CAD build for the part. Positions are in the model's coordinates, mm. A direction names the side the tool comes from. Round coordinates to 2 decimals unless told otherwise and drop trailing zeros. Order: outer loops, then holes, each group sorted by start corner. A loop starts at its lowest first (then second) coordinate and runs counter-clockwise, first axis right, second up. Notation, with made-up numbers: M 66,34 L 97,34 A12 cw 97,40 Z; hole C 54.5,8.5 d5. An arc over 180 degrees is marked long. Put each result on its own line as item: value.
```python
from build123d import *

# Parameters (mm, degrees)
BOSS_EXTRUDE1_DEPTH = 127
SKETCH3_R           = 3.175
CUT_EXTRUDE1_DEPTH  = 145.837083045
SKETCH4_R           = 2.5
SKETCH4_R_2         = 2.413
SKETCH4_R_3         = 3.175
SKETCH4_R_4         = 4
CUT_EXTRUDE2_DEPTH  = 146.911891222


with BuildPart() as part:
    # Sketch2 → Boss-Extrude1 (new body)
    with BuildSketch(Plane.XY):
        Polygon((0, 0), (0, 50.8), (3.175, 50.8), (3.175, 3.175), (50.8, 3.175), (50.8, 0), align=None)
    extrude(amount=BOSS_EXTRUDE1_DEPTH)

    # Sketch3 → Cut-Extrude1 (cut, through all)
    with BuildSketch(Plane(origin=(0, 3.175, 0), x_dir=(1, 0, 0), z_dir=(0, 1, 0))):
        with Locations(Location((17.0942, -9.525, 0), (0, 0, 180))):
            Circle(SKETCH3_R)
        with Locations(Location((17.0942, -78.624999976, 0), (0, 0, 180))):
            Circle(SKETCH3_R)
        with Locations(Location((17.0942, -117.475, 0), (0, 0, 180))):
            Circle(SKETCH3_R)
    extrude(amount=-CUT_EXTRUDE1_DEPTH, mode=Mode.SUBTRACT)

    # Sketch4 → Cut-Extrude2 (cut, through all)
    with BuildSketch(Plane.ZY):
        with Locations((20.5994, 14.155)):
            Circle(SKETCH4_R)
        with Locations((9.525, 41.275)):
            Circle(SKETCH4_R_2)
        with Locations((67.7394, 14.155)):
            Circle(SKETCH4_R)
        with Locations((78.625, 41.275)):
            Circle(SKETCH4_R_2)
        with Locations((44.1706, 37.725)):
            Circle(SKETCH4_R_3)
        with Locations((94.9706, 37.725)):
            Circle(SKETCH4_R_4)
    extrude(amount=-CUT_EXTRUDE2_DEPTH, mode=Mode.SUBTRACT)


solid = part.part
```
Item 1: Probe line 1 along X through (y, z) = (16.5, 40) (3 decimals). List the from-to ranges inside material, lowest first. Write a range as [from, to].
Answers below:
line 1: [0, 3.175]
Item 2: Band-saw the part on C-C on y = 21.5. Give the cut face in (x, z) (3 decimals), and give its area (3 significant figures).
Answers below:
outline: M 0,0 L 3.175,0 L 3.175,127 L 0,127 Z
area: 403 mm²
Item 3: Band-saw the part on A-A on z = 95. Give the cut face in (x, y) (3 decimals), and give its area (3 significant figures).
Answers below:
outline: M 0,0 L 50.8,0 L 50.8,3.175 L 3.175,3.175 L 3.175,33.725 L 0,33.725 Z; M 0,41.725 L 3.175,41.725 L 3.175,50.8 L 0,50.8 Z
area: 287 mm²
Item 4: Mould opens along Y. For faces 1 (the flat face through (27, 3.175, 63)), 2 (the cylindrical face through (1.565, 16.263, 21.943)), 3 (the cylindrical face through (17.508, 1.61, 12.673)), 4 (the cylindrical face through (1.57, 43.31, 10.82)) say: pulls with the +Y half, pulls with the -Y half, needs draft (parallel to the pull), parting line crosses it, or undercut.
Answers below:
face 1: pulls with the +Y half
face 2: undercut
face 3: needs draft
face 4: undercut
Item 5: Band-saw the part on B-B on x = 18. Give the cut face in (y, z) (3 decimals), and give its area (3 significant figures).
Answers below:
outline: M 0,0 L 3.175,0 L 3.175,6.482 L 0,6.482 Z; M 0,12.568 L 3.175,12.568 L 3.175,75.582 L 0,75.582 Z; M 0,81.668 L 3.175,81.668 L 3.175,114.432 L 0,114.432 Z; M 0,120.518 L 3.175,120.518 L 3.175,127 L 0,127 Z
area: 345 mm²
Item 6: Pin check, flat tips, straight feed: P1, Ø4, axis at y = 37.72, z = 44.17, coming from the -X side; P2, Ø2, axis at x = 20, z = 96, coming from the +Y side (3 decimals); P3, Ø5.5, axis at y = 41.275, z = 78.625, coming from the +X side (3 decimals). Stop position of each tip, or through.
Answers below:
P1: through
P2: y = 3.175
P3: x = 3.175
Item 7: Tool access for faces 5 (the flat face through (26, 0, 63)), 6 (the flat face through (3.175, 27, 63)): list every direction of +Z, -Z, +X, -X, +Y, -Y with a clear straight run to the whole face (end or side of a thin tool).
Answers below:
face 5: +Z, -Z, +X, -X, -Y
face 6: +Z, -Z, +X, +Y
